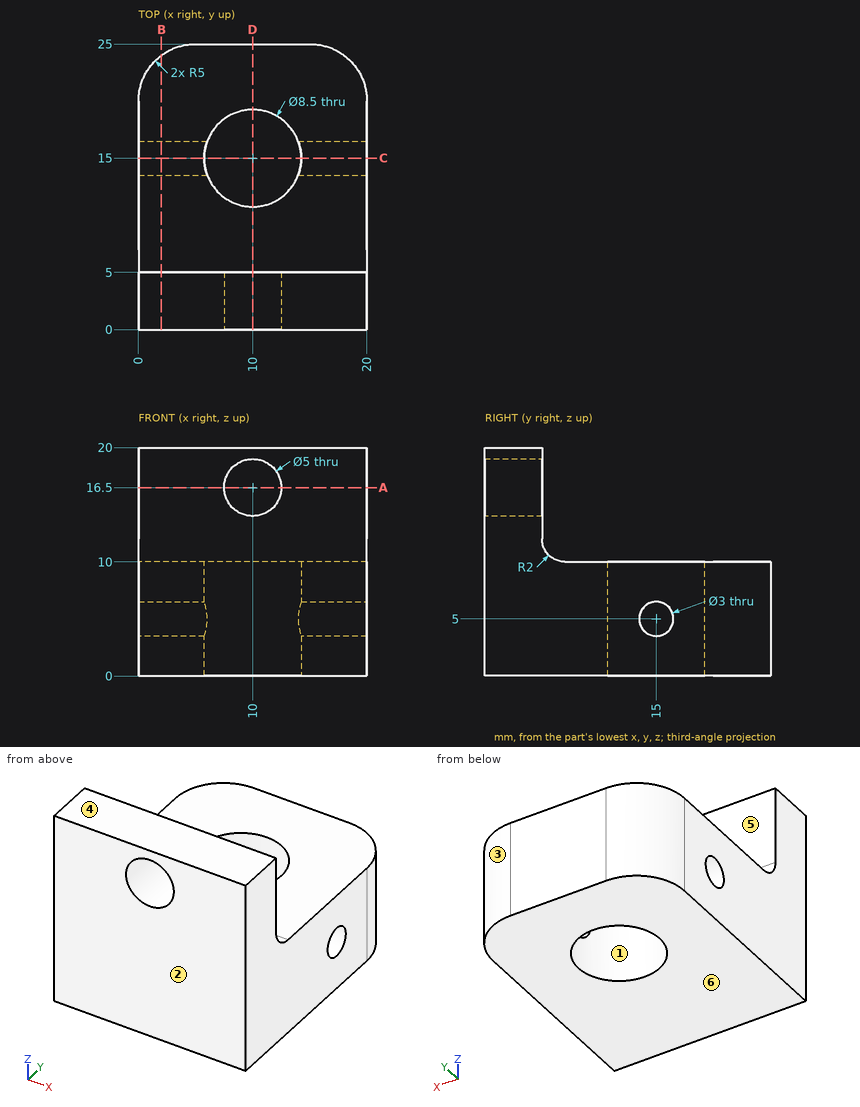
Source: three-view drawing plus pictorial views. Frame: mm from the lowest corner of the part. A direction names the side the tool comes from. Give positions to 0.01 mm unless a question says otherwise; leave off trailing zeros. Loops run counter-clockwise (first coordinate to the right, second up) from the corner with the lowest first, then second, coordinate; pieces in that order, holes last. Notation, with made-up numbers: M -34.75,9.25 L 22.25,9.25 A23 cw 22.25,36.25 Z; hole C 47.5,41.25 d9. An arc over 180 degrees is marked long. Put each result on its own line as item: value.
Q1. Section A-A (z = 16.5). Return the cut outline in (x, y).
Response values:
outline: M 0,0 L 7.5,0 L 7.5,5 L 0,5 Z; M 12.5,0 L 20,0 L 20,5 L 12.5,5 Z
Q2. Pin query (flat end, axial travel): P1, Ø2, axis at x = 11, y = 21.5, coming from the +Z side; P2, Ø8, axis at x = 5, z = 6, coming from the -Y side; P3, Ø2.5, axis at x = 9, z = 14.5, coming from the +Y side. Return the tip coordinate at first contact, or that it passes through.
Response values:
P1: stops at z = 10
P2: stops at y = 0
P3: stops at y = 5
Q3. Section B-B (x = 2). Return the cut outline in (y, z), and give its area (3 significant figures).
Response values:
outline: M 0,0 L 24,0 L 24,10 L 7,10 A2 cw 5,12 L 5,20 L 0,20 Z; hole C 15,5 d3
area: 284 mm²
Q4. Section C-C (y = 15). Return the cut outline in (x, z).
Response values:
outline: M 0,0 L 5.75,0 L 5.75,3.5 L 0,3.5 Z; M 0,6.5 L 5.75,6.5 L 5.75,10 L 0,10 Z; M 14.25,0 L 20,0 L 20,3.5 L 14.25,3.5 Z; M 14.25,6.5 L 20,6.5 L 20,10 L 14.25,10 Z
Q5. Section D-D (x = 10). Return the cut outline in (y, z).
Response values:
outline: M 0,0 L 10.75,0 L 10.75,10 L 7,10 A2 cw 5,12 L 5,14 L 0,14 Z; M 0,19 L 5,19 L 5,20 L 0,20 Z; M 19.25,0 L 25,0 L 25,10 L 19.25,10 Z
Q6. Line query: probe 1 along Y at (x, z) = (10, 4.75); probe 2 along Z at (x, y) = (18, 15); probe 3 along X at (y, z) = (1.4, 16.5). Output: solid intervals per line, ascending. Write a range as [from, to].
Response values:
probe 1: y = [0, 10.75], [19.25, 25]
probe 2: z = [0, 3.5], [6.5, 10]
probe 3: x = [0, 7.5], [12.5, 20]
Q7. Reachability of the marked faces 5 and 6 from +Z, -Z, +X, -X, +Y, -Y: full face, straight path, thin tool, end or side. Return the list, or none.
Response values:
face 5: +Z, +X, -X, +Y
face 6: -Z, +X, -X, +Y, -Y
Q8. Mould query, pull axis Y, two halves, no side actions, for the marked faces 1, 2, 3 and 4. Classes: released by +Y, released by -Y, zero draft, split by the parting line, or undercut.
Response values:
face 1: undercut
face 2: released by -Y
face 3: released by +Y
face 4: zero draft
